from build123d import *

# Parameters (mm, degrees)
F0_W     = 63.5
F0_H     = 79.375
F1_DEPTH = 53.975
F2_R     = 1.5875
F3_DEPTH = 3.175
F4_R     = 7.9375
F5_DEPTH = 1.5875
F6_R     = 4.7625
F7_DEPTH = 12.7


with BuildPart() as f1:
    # F0 (on Front) → F1 (new body)
    with BuildSketch(Plane.XZ):
        Rectangle(F0_W, F0_H)
    extrude(amount=F1_DEPTH)

    # F2 (on face) → F3 (join)
    with BuildSketch(Plane.YZ.offset(31.75)):
        with Locations((-40.005, 23.8125)):
            Circle(F2_R)
        with Locations((-40.005, -26.9875)):
            Circle(F2_R)
        with Locations((-14.605, 23.8125)):
            Circle(F2_R)
        with Locations((-14.605, -26.9875)):
            Circle(F2_R)
    extrude(amount=F3_DEPTH)

    # F4 (on face) → F5 (join)
    with BuildSketch(Plane.YZ.offset(34.925)):
        with Locations((-40.005, 23.8125)):
            Circle(F4_R)
        with Locations((-14.605, 23.8125)):
            Circle(F4_R)
        with Locations((-40.005, -26.9875)):
            Circle(F4_R)
        with Locations((-14.605, -26.9875)):
            Circle(F4_R)
    extrude(amount=F5_DEPTH)

    # F6 (on face) → F7 (join)
    with BuildSketch(Plane(origin=(-31.75, 0, 0), x_dir=(0, -1, 0), z_dir=(-1, 0, 0))):
        with Locations((26.9875, -7.9375)):
            Circle(F6_R)
    extrude(amount=F7_DEPTH)


solid = f1.part
Model file for the job. Use its own axes, mm. A direction names the side the tool comes from. Give positions to 0.01 mm unless a question says otherwise; leave off trailing zeros. Loops run counter-clockwise (first coordinate to the right, second up) from the corner with the lowest first, then second, coordinate; pieces in that order, holes last.
Item 1: Slice it at C-C (z = -5.5). Write the cut outline in (x, y) (3 decimals), plus the area to 3 significant figures.
Check values:
outline: (-44.45, -31.079) - (-31.75, -31.079) - (-31.75, -53.975) - (31.75, -53.975) - (31.75, 0) - (-31.75, 0) - (-31.75, -22.896) - (-44.45, -22.896) - close
area: 3,530 mm2
Item 2: Drill centre lines: line 1 along X through (y, z) = (-2, -29); line 2 along X through (y, z) = (-29, -7.5). Where is each one in solid material? Low to high.
Check values:
line 1: x = -31.75 to 31.75
line 2: x = -44.45 to 31.75
Item 3: Mould opens along Z. For faces 1 (the face through (0, -27, -39.688)), 2 (the face through (35.708, -7.034, 26.197)), 3 (the face through (36.512, -15, 24)), 4 (the face through (-38.01, -22.23, -7.73)) say: +Z half, -Z half, draft (parallel to the pull), parting line (faces both ways), or undercut.
Check values:
face 1: -Z half
face 2: undercut
face 3: draft
face 4: parting line
Item 4: Slice it at D-D (y = -26). Write the cut outline in (x, z).
Check values:
outline: (-44.45, -12.6) - (-31.75, -12.6) - (-31.75, -39.69) - (31.75, -39.69) - (31.75, 39.69) - (-31.75, 39.69) - (-31.75, -3.28) - (-44.45, -3.28) - close
Item 5: Slice it at A-A (z = -22.5). Give the number of separate pieces and of enclosed holes in the cut face, plus the area to 3 significant figures.
Check values:
separate pieces: 3
enclosed holes: 0
area: 3,470 mm2
Item 6: Drop a flat-ended pin along its axis: P1, Ø17.5, axis at y = -36, z = -25, coming from the -X side. Give the stop position or say it passes through.
Check values:
P1: stops at x = -31.75
Item 7: Which spindle directions (+Z, -Z, +X, -X, +Y, -Y) get a long thin tool onto all of the face, cutting with end or side? Do faces 5 (the face through (35.71, -46.3, -31.82)), 6 (the face through (0, -53.975, 1)), 7 (the face through (33.315, -14.949, 22.263)). Say none if no direction does.
Check values:
face 5: +X
face 6: +Z, -Z, +X, -X, -Y
face 7: none
